```python
from build123d import *

# Parameters (mm, degrees)
SKETCH_1_W           = 75
SKETCH_1_H           = 80
EXTRUDE_1_DEPTH      = 60
CUT_EXTRUDE_2_DEPTH  = 70
SKETCH_2_4_W         = 26.5
SKETCH_2_4_H         = 27
CUT_EXTRUDE_3_DEPTH  = 70
SKETCH_2_5_W         = 21
SKETCH_2_5_H         = 26
SKETCH_2_5_W_2       = 2
SKETCH_2_5_H_2       = 2.25
CUT_EXTRUDE_4_DEPTH  = 50
SKETCH_2_W           = 3
SKETCH_2_H           = 5
SKETCH_2_W_2         = 49
SKETCH_2_H_2         = 17
CUT_EXTRUDE_5_DEPTH  = 70
SKETCH_4_W           = 2
SKETCH_4_H           = 75
CUT_EXTRUDE_6_DEPTH  = 3
SKETCH_6_W           = 25
SKETCH_6_H           = 3
CUT_EXTRUDE_7_DEPTH  = 81
SKETCH_7_W           = 3
SKETCH_7_H           = 2
CUT_EXTRUDE_8_DEPTH  = 3
SKETCH_9_W           = 60
SKETCH_9_H           = 80
CUT_EXTRUDE_11_DEPTH = 4
SKETCH_10_W          = 2
SKETCH_10_H          = 75
CUT_EXTRUDE_12_DEPTH = 3
SKETCH_8_W           = 8
SKETCH_8_H           = 12
SKETCH_8_W_2         = 7.2
SKETCH_8_H_2         = 20
CUT_EXTRUDE_13_DEPTH = 70


with BuildPart() as part:
    # Sketch 1 → Extrude 1 (new body)
    with BuildSketch(Plane.XY):
        with Locations((-39.564393939, 27.339015152)):
            Rectangle(SKETCH_1_W, SKETCH_1_H)
    extrude(amount=EXTRUDE_1_DEPTH)

    # Sketch 2_3 → Cut-Extrude 2 (cut)
    with BuildSketch(Plane(origin=(-2.064393939, 0, 0), x_dir=(0, 0, -1), z_dir=(1, 0, 0))):
        Polygon((-54, 62.339015152), (-54, 42.339015152), (-26.2, 42.339015152), (-26.2, 57.339015152), (-15.2, 57.339015152), (-15.2, 41.339015152), (-10.2, 41.339015152), (-10.2, 62.339015152), align=None)
    extrude(amount=-CUT_EXTRUDE_2_DEPTH, mode=Mode.SUBTRACT)

    # Sketch 2_4 → Cut-Extrude 3 (cut)
    with BuildSketch(Plane(origin=(-2.064393939, 0, 0), x_dir=(0, 0, -1), z_dir=(1, 0, 0))):
        with Locations((-40.75, 28.839015152)):
            Rectangle(SKETCH_2_4_W, SKETCH_2_4_H)
    extrude(amount=-CUT_EXTRUDE_3_DEPTH, mode=Mode.SUBTRACT)

    # Sketch 2_5 → Cut-Extrude 4 (cut)
    with BuildSketch(Plane(origin=(-2.064393939, 0, 0), x_dir=(0, 0, -1), z_dir=(1, 0, 0))):
        with Locations((-13.5, 28.339015152)):
            Rectangle(SKETCH_2_5_W, SKETCH_2_5_H)
        with Locations((-25, 16.464015152)):
            Rectangle(SKETCH_2_5_W_2, SKETCH_2_5_H_2)
        with Locations((-2, 16.464015152)):
            Rectangle(SKETCH_2_5_W_2, SKETCH_2_5_H_2)
    extrude(amount=-CUT_EXTRUDE_4_DEPTH, mode=Mode.SUBTRACT)

    # Sketch 2 → Cut-Extrude 5 (cut)
    with BuildSketch(Plane(origin=(-2.064393939, 0, 0), x_dir=(0, 0, -1), z_dir=(1, 0, 0))):
        with Locations((-39.306060925, 12.839015152)):
            Rectangle(SKETCH_2_W, SKETCH_2_H)
        with Locations((-27.5, 1.839015152)):
            Rectangle(SKETCH_2_W_2, SKETCH_2_H_2)
    extrude(amount=-CUT_EXTRUDE_5_DEPTH, mode=Mode.SUBTRACT)

    # Sketch 4 → Cut-Extrude 6 (cut)
    with BuildSketch(Plane(origin=(0, 0, 0), x_dir=(-1, 0, 0), z_dir=(0, 0, -1))):
        with Locations((5.064393939, 26.839015152)):
            Rectangle(SKETCH_4_W, SKETCH_4_H)
    extrude(amount=-CUT_EXTRUDE_6_DEPTH, mode=Mode.SUBTRACT)

    # Sketch 6 → Cut-Extrude 7 (cut, through all)
    with BuildSketch(Plane(origin=(0, 67.339015152, 0), x_dir=(1, 0, 0), z_dir=(0, 1, 0))):
        with Locations((-39.564393939, -57)):
            Rectangle(SKETCH_6_W, SKETCH_6_H)
    extrude(amount=-CUT_EXTRUDE_7_DEPTH, mode=Mode.SUBTRACT)

    # Sketch 7 → Cut-Extrude 8 (cut)
    with BuildSketch(Plane(origin=(-52.064393939, 0, 0), x_dir=(0, 0, -1), z_dir=(1, 0, 0))):
        with Locations((-13.75, 16.339015152)):
            Rectangle(SKETCH_7_W, SKETCH_7_H)
    extrude(amount=-CUT_EXTRUDE_8_DEPTH, mode=Mode.SUBTRACT)

    # Sketch 9 → Cut-Extrude 11 (cut)
    with BuildSketch(Plane.ZY.offset(77.064393939)):
        with Locations((30, 27.339015152)):
            Rectangle(SKETCH_9_W, SKETCH_9_H)
    extrude(amount=-CUT_EXTRUDE_11_DEPTH, mode=Mode.SUBTRACT)

    # Sketch 10 → Cut-Extrude 12 (cut)
    with BuildSketch(Plane.XY.offset(60)):
        with Locations((-5.064393939, 26.839015152)):
            Rectangle(SKETCH_10_W, SKETCH_10_H)
    extrude(amount=-CUT_EXTRUDE_12_DEPTH, mode=Mode.SUBTRACT)

    # Sketch 8 → Cut-Extrude 13 (cut)
    with BuildSketch(Plane(origin=(-2.064393939, 0, 0), x_dir=(0, 0, -1), z_dir=(1, 0, 0))):
        with Locations((-20.7, 49.839015152)):
            Rectangle(SKETCH_8_W, SKETCH_8_H)
        with Locations((-5.1, 54.339015152)):
            Rectangle(SKETCH_8_W_2, SKETCH_8_H_2)
    extrude(amount=-CUT_EXTRUDE_13_DEPTH, mode=Mode.SUBTRACT)


solid = part.part
```
Geometry check sheet. Reference: the model listing, model coordinates, mm. A direction names the side the tool comes from. Give positions to 0.01 mm unless a question says otherwise; leave off trailing zeros. Order: outer loops, then holes, each group sorted by start corner. A loop starts at its lowest first (then second) coordinate and runs counter-clockwise, first axis right, second up.
1. Access from +Z, -Z, +X, -X, +Y, -Y to the whole of each face (thin tool, end or side, straight path). Record for faces 3 (the face through (-6.064, 26, 1)), 4 (the face through (-28, 15.339, 14)), 5 (the face through (-5, -10.661, 59)).
2. Section check A-A, the plane y = 6.5. Enter the section's corners in (x, z).
3. Section check B-B, the plane x = -62.5. Give the number of separate pieces and of enclosed holes in the cut face, and give its area (3 significant figures).
4. Gauge pin test, flat ends, axial feed: pin 1 Ø8 at (y, z) = (26.5, 22) entering from +X; pin 2 Ø0.6 at (y, z) = (16, 14) entering from +X. Record the tip position at first contact, or that the pin passes through.
5. Release check for a two-part mould opening along X. For faces 1 (the face through (-5, -10.661, 1)), 2 (the face through (-37, 57.339, 21)) record: pulls with the +X half, pulls with the -X half, needs draft (parallel to the pull), parting line crosses it, or undercut.
6. Section check C-C, the plane y = 35. Enter the section's corners in (x, z), and give its area (3 significant figures).
7. Section check D-D, the plane z = 34. Enter the section's corners in (x, y), and give its area (3 significant figures).
8. Thickness scan on L1, parallel to Y at x = -62, z = 17.5; L2, parallel to Z at x = -32, y = 33; L3, parallel to Y at x = -44, z = 46. Record the ranges inside material, lowest first.
Values follow:
1. face 3: -Z
1. face 4: +X
1. face 5: +Z
2. outline: (-73.06, 0) - (-6.06, 0) - (-6.06, 3) - (-72.06, 3) - (-72.06, 52) - (-2.06, 52) - (-2.06, 60) - (-4.06, 60) - (-4.06, 57) - (-6.06, 57) - (-6.06, 60) - (-73.06, 60) - close; (-4.06, 0) - (-2.06, 0) - (-2.06, 3) - (-4.06, 3) - close; hole (-52.06, 55.5) - (-27.06, 55.5) - (-27.06, 58.5) - (-52.06, 58.5) - close
3. separate pieces: 1
3. enclosed holes: 3
3. area: 2,280 mm2
4. pin 1: stops at x = -2.06
4. pin 2: stops at x = -55.06
5. face 1: undercut
5. face 2: needs draft
6. outline: (-73.06, 0) - (-6.06, 0) - (-6.06, 3) - (-52.06, 3) - (-52.06, 24) - (-2.06, 24) - (-2.06, 27.5) - (-72.06, 27.5) - (-72.06, 54) - (-2.06, 54) - (-2.06, 60) - (-4.06, 60) - (-4.06, 57) - (-6.06, 57) - (-6.06, 60) - (-73.06, 60) - close; (-4.06, 0) - (-2.06, 0) - (-2.06, 3) - (-4.06, 3) - close; hole (-52.06, 55.5) - (-27.06, 55.5) - (-27.06, 58.5) - (-52.06, 58.5) - close
6. area: 1,270 mm2
7. outline: (-73.06, -12.66) - (-2.06, -12.66) - (-2.06, -6.66) - (-72.06, -6.66) - (-72.06, 10.34) - (-2.06, 10.34) - (-2.06, 15.34) - (-72.06, 15.34) - (-72.06, 62.34) - (-2.06, 62.34) - (-2.06, 67.34) - (-73.06, 67.34) - close
7. area: 1,200 mm2
8. L1: y = -12.66 to -6.66, 10.34 to 43.84, 55.84 to 57.34, 62.34 to 67.34
8. L2: z = 0 to 3, 24 to 27.5, 54 to 55.5, 58.5 to 60
8. L3: y = -12.66 to -6.66, 10.34 to 15.34, 62.34 to 67.34
